Source: CAD feature listing. Evaluate the final solid. Frame: model axes, mm. Face numbers are marked on the shaded views. A direction names the side the tool comes from. Round coordinates to 2 decimals unless told otherwise and drop trailing zeros. Write each loop counter-clockwise with the first axis right and the second up, starting at its lowest first coordinate (ties: lowest second). Pieces come first, ordered by that corner, then holes.
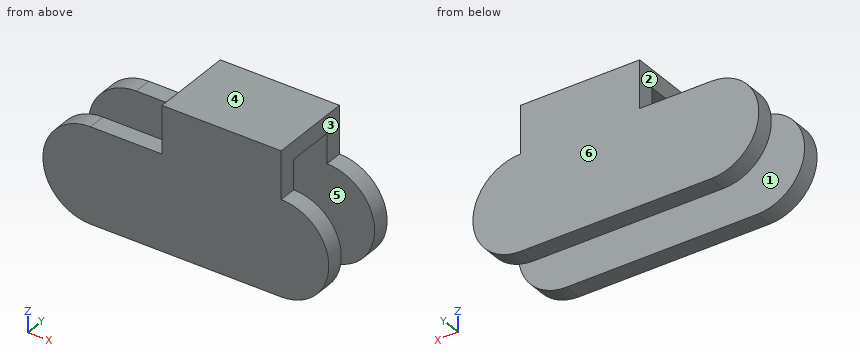
from build123d import *

# Parameters (mm, degrees)
F0_R     = 3
F1_DEPTH = 14
F2_T     = -3


with BuildPart() as f1:
    # F0 (on Front) → F1 (new body)
    with BuildSketch(Plane.XZ):
        with BuildLine():
            ThreePointArc((-16, 8), (-24, 0), (-16, -8))
            Line((-16, -8), (16, -8))
            ThreePointArc((16, -8), (24, 0), (16, 8))
            Line((16, 8), (16, 16))
            Line((16, 16), (-4, 16))
            Line((-4, 16), (-4, 8))
            Line((-4, 8), (-16, 8))
        make_face()
        with Locations((-16, 0)):
            Circle(F0_R, mode=Mode.SUBTRACT)
        with Locations((16, 0)):
            Circle(F0_R, mode=Mode.SUBTRACT)
        with Locations((-16, 0)):
            Circle(F0_R)
        with Locations((16, 0)):
            Circle(F0_R)
    extrude(amount=-F1_DEPTH)

    # F2
    f2_openings = [f1.faces().sort_by_distance(p)[0] for p in [
        (-10, 7, 8),
        (-4, 7, 12),
        (24, 7, 0),
        (-24, 7, 0),
        (0, 7, -8),
        (16, 7, 12),
    ]]
    offset(amount=F2_T, openings=f2_openings)


solid = f1.part
1) Material intervals for line 1 (Y direction, x = -5.5, z = -4.75); line 2 (Z direction, x = -10.5, y = 12.75); line 3 (Z direction, x = 8.5, y = 10.25), sorted ascending.
Taken from the geometry:
line 1: y = 0 to 3, 11 to 14
line 2: z = -8 to 8
line 3: z = 13 to 16
2) Section query B-B on x = -11. Return the cut outline in (y, z), then the cut area to 3 significant figures.
Taken from the geometry:
outline: (0, -8) - (3, -8) - (3, 8) - (0, 8) - close; (11, -8) - (14, -8) - (14, 8) - (11, 8) - close
area: 96.0 mm2
3) Contact query for flat-ended pins moving along their axis: P1, Ø6.5, axis at y = 6, z = 12.5, coming from the +X side; P2, Ø5, axis at y = 12, z = -5, coming from the -X side; P3, Ø4, axis at x = 5, y = 8.5, coming from the -Z side; P4, Ø6.5, axis at x = 4.5, z = 1.5, coming from the -Y side. Output: stop coordinate, or through.
Taken from the geometry:
P1: stops at x = 16
P2: stops at x = -23.6
P3: stops at z = 13
P4: stops at y = 0
4) Pull-direction query (Y, two-part tool) for the marked faces 4, 5 and 6; classes: released by +Y, released by -Y, zero draft, split by the parting line, or undercut.
Taken from the geometry:
face 4: zero draft
face 5: undercut
face 6: released by +Y
5) Section query D-D on y = 9.5. Return the cut outline in (x, z), then the cut area to 3 significant figures.
Taken from the geometry:
outline: (-4, 13) - (16, 13) - (16, 16) - (-4, 16) - close
area: 60.0 mm2
6) Section query C-C on x = 13.5. Return the cut outline in (y, z), then the cut area to 3 significant figures.
Taken from the geometry:
outline: (0, -8) - (3, -8) - (3, 13) - (11, 13) - (11, -8) - (14, -8) - (14, 16) - (0, 16) - close
area: 168 mm2
7) Section query A-A on z = 0. Return the cut outline in (x, y).
Taken from the geometry:
outline: (-24, 0) - (24, 0) - (24, 3) - (-24, 3) - close; (-24, 11) - (24, 11) - (24, 14) - (-24, 14) - close
8) Reachability of the marked faces 1, 2 and 3 from +Z, -Z, +X, -X, +Y, -Y: full face, straight path, thin tool, end or side. Return the list, or none.
Taken from the geometry:
face 1: -Z, +X, -X
face 2: +Z, -X, +Y, -Y
face 3: +Z, +X, +Y, -Y
